Autodesk Inventor part; units mm, degrees
ref_plane "YZ Plane" through (0, 0, 0) normal (1, 0, 0) x (0, 1, 0)
ref_plane "XZ Plane" through (0, 0, 0) normal (0, 1, 0) x (-1, 0, 0)
ref_plane "XY Plane" through (0, 0, 0) normal (0, 0, 1) x (1, 0, 0)
sketch "Sketch1" plane through (0, 0, 0) normal (0, 0, 1) x (1, 0, 0)
  line L0 (0, 0) -> (1841.5, 0)
  line L1 (1841.5, 0) -> (1841.5, 812.8)
  line L2 (1841.5, 812.8) -> (1606.55, 812.8)
  line L3 (1606.55, 812.8) -> (1606.55, 660.4)
  line L4 (1606.55, 660.4) -> (234.95, 660.4)
  line L5 (234.95, 660.4) -> (234.95, 812.8)
  line L6 (234.95, 812.8) -> (0, 812.8)
  line L7 (0, 812.8) -> (0, 0)
  dimension "d0" = 1841.5
  dimension "d1" = 812.8
  dimension "d2" = 234.95
  dimension "d3" = 152.4
  dimension "d4" = 234.95
  dimension "d5" = 152.4
extrude "Extrusion1" add sketch "Sketch1" against normal blind 3.175
equation "\"d4\" = d2"
equation "\"d5\" = d3"
properties part number "GE-13013B" material "Polycarbonate, Clear"
Input: part model. Units: mm. Frame: model coordinates. Coordinates: 2 decimals unless noted, no trailing zeros. Loops run counter-clockwise (first coordinate to the right, second up) from the corner with the lowest first, then second, coordinate; pieces in that order, holes last.
Q1. Contact query for a flat-ended pin moving along its axis: pin 1 (1 mm diameter, centred on x = 373, z = -2.5, fed in from +Y). Output: stop coordinate, or through.
Q2. Cut plane C-C (x = 602.5). Output: boundary loops of the cut face in (y, z) (3 decimals).
Q3. Cut plane B-B (z = -0.55). Output: boundary loops of the cut face in (x, y), then the cut area to 3 significant figures.
Q4. Material intervals for line 1 (Y direction, x = 389.5, z = -1.7); line 2 (X direction, y = 736.5, z = -1.1), sorted ascending.
Q5. Cut plane A-A (y = 700). Output: boundary loops of the cut face in (x, z) (3 decimals).
Working result:
1. pin 1: stops at y = 660.4
2. outline: (0, -3.175) - (660.4, -3.175) - (660.4, 0) - (0, 0) - close
3. outline: (0, 0) - (1841.5, 0) - (1841.5, 812.8) - (1606.55, 812.8) - (1606.55, 660.4) - (234.95, 660.4) - (234.95, 812.8) - (0, 812.8) - close
3. area: 1,290,000 mm2
4. line 1: y = 0 to 660.4
4. line 2: x = 0 to 234.95, 1606.55 to 1841.5
5. outline: (0, -3.175) - (234.95, -3.175) - (234.95, 0) - (0, 0) - close; (1606.55, -3.175) - (1841.5, -3.175) - (1841.5, 0) - (1606.55, 0) - close
